from build123d import *

# Parameters (mm, degrees)
F0_W     = 207.3402
F0_H     = 304.8
F1_DEPTH = 34.29
F2_DEPTH = 12.7
F3_R     = 5.08
F4_R     = 7.14375
F4_R_2   = 9.331431
F5_DEPTH = 34.291


with BuildPart() as f1:
    # F0 (on Top) → F1 (new body)
    with BuildSketch(Plane.XY):
        Rectangle(F0_W, F0_H)
    extrude(amount=F1_DEPTH)

    # F0 (on Top) → F2 (join)
    with BuildSketch(Plane.XY):
        Polygon((-103.6701, -152.4), (-103.6701, 152.4), (-167.1701, 152.4), (-167.1701, -153.244078), (-103.6701, -153.244078), align=None)
        Polygon((167.1701, 152.4), (103.6701, 152.4), (103.6701, -152.4), (103.6701, -152.423114), (167.1701, -152.423114), align=None)
    extrude(amount=F2_DEPTH)

    # F3
    f3_edges = [f1.edges().sort_by_distance(p)[0] for p in [
        (-167.1701, -0.422039, 12.7),
        (-103.6701, 0, 34.29),
        (103.6701, 0, 34.29),
        (167.1701, -0.011557, 12.7),
    ]]
    fillet(f3_edges, radius=F3_R)

    # F4 (on face) → F5 (cut, through all)
    with BuildSketch(Plane.XY.offset(34.29)):
        with Locations((-133.920491, 121.190689)):
            Circle(F4_R)
        with Locations((-75.377315, 121.190689)):
            Circle(F4_R)
        with Locations((69.863357, 121.190689)):
            Circle(F4_R)
        with Locations((132.428586, 121.190689)):
            Circle(F4_R)
        with Locations((132.428586, -132.809311)):
            Circle(F4_R_2)
        with Locations((69.863357, -132.809311)):
            Circle(F4_R_2)
        with Locations((-75.377315, -132.809311)):
            Circle(F4_R_2)
        with Locations((-133.920491, -132.809311)):
            Circle(F4_R_2)
    extrude(amount=-F5_DEPTH, mode=Mode.SUBTRACT)


solid = f1.part
Could you check a few things on this model? Use its own coordinates, in mm. A direction names the side the tool comes from. Round coordinates to 2 decimals unless told otherwise and drop trailing zeros. Order: outer loops, then holes, each group sorted by start corner. A loop starts at its lowest first (then second) coordinate and runs counter-clockwise, first axis right, second up.
Q1. Which directions (+Z, -Z, +X, -X, +Y, -Y) give clear straight access to the entire face, cutting with the end or side of a thin tool? Please do faces 1 (the face through (-167.17, 2, 4)), 2 (the face through (-1, -152.4, 17)), 3 (the face through (-76.592, -123.557, 17.385)), 4 (the face through (132, 2, 12.7)), 5 (the face through (-103.67, -2, 21)).
Geometry says:
face 1: +Z, -Z, -X, +Y, -Y
face 2: +Z, -Z, +X, -Y
face 3: +Z, -Z
face 4: +Z, +X, +Y, -Y
face 5: +Z, -X, +Y, -Y
Q2. I'm going to push flat-ended pins straight in: P1, Ø5, axis at y = 42, z = 19.5, coming from the +X side; P2, Ø23, axis at x = -133.92, y = 121.19, coming from the +Z side; P3, Ø0.9, axis at y = -153, z = 8.5, coming from the +X side; P4, Ø17, axis at x = 132.43, y = -132.81, coming from the -Z side. Where does each tip first touch, or does it pass through?
Geometry says:
P1: stops at x = 103.67
P2: stops at z = 12.7
P3: stops at x = -103.67
P4: passes through
Q3. Please list where these lines run through material, in increasing order: probe 1 along Y at (x, z) = (-77.5, 17); probe 2 along Y at (x, z) = (-37, 7.5); probe 3 along X at (y, z) = (-8.5, 22).
Geometry says:
probe 1: y = -152.4 to -141.9, -123.72 to 114.37, 128.01 to 152.4
probe 2: y = -152.4 to 152.4
probe 3: x = -103.67 to 103.67
Q4. Thinking about a two-plate mould opening in Y: for faces 6 (the face through (-135.135, -123.557, 6.439)), 7 (the face through (-136, -153.244, 6)), 8 (the face through (-2, 2, 0)), which applies, released by +Y, released by -Y, zero draft, split by the parting line, or undercut?
Geometry says:
face 6: undercut
face 7: released by -Y
face 8: zero draft
Q5. Imagine slicing it at A-A, the plane x = 134.5. List the corners of the cut face in (y, z) for me, then the cut area to 3 significant figures.
Geometry says:
outline: (-152.42, 0) - (-141.91, 0) - (-141.91, 12.7) - (-152.42, 12.7) - close; (-123.71, 0) - (114.35, 0) - (114.35, 12.7) - (-123.71, 12.7) - close; (128.03, 0) - (152.4, 0) - (152.4, 12.7) - (128.03, 12.7) - close
area: 3,470 mm2
Q6. Imagine slicing it at B-B, the plane y = 95. List the corners of the cut face in (x, z) for me, then the cut area to 3 significant figures.
Geometry says:
outline: (-167.17, 0) - (167.17, 0) - (167.17, 7.62) arc R5.08 ccw to (162.09, 12.7) - (103.67, 12.7) - (103.67, 29.21) arc R5.08 ccw to (98.59, 34.29) - (-98.59, 34.29) arc R5.08 ccw to (-103.67, 29.21) - (-103.67, 12.7) - (-162.09, 12.7) arc R5.08 ccw to (-167.17, 7.62) - close
area: 8,700 mm2
Q7. Imagine slicing it at C-C, the plane z = 23.5. List the corners of the cut face in (x, y) for me, then the cut area to 3 significant figures.
Geometry says:
outline: (-103.67, -152.4) - (103.67, -152.4) - (103.67, 152.4) - (-103.67, 152.4) - close; hole circle Ø18.66 at (-75.38, -132.81); hole circle Ø14.29 at (-75.38, 121.19); hole circle Ø18.66 at (69.86, -132.81); hole circle Ø14.29 at (69.86, 121.19)
area: 62,300 mm2
